Geometry: see drawing. Coordinates: mm, zero at the bounding-box minimum. Give positions to 0.01 mm unless a question says otherwise; leave off trailing zeros. Loops run counter-clockwise (first coordinate to the right, second up) from the corner with the lowest first, then second, coordinate; pieces in that order, holes last. Notation, with made-up numbers: (-17.75, -27) -> (40.25, -27) arc R15 ccw to (40.25, -22) -> close; hole circle Ø8 at (17.5, -20.75). An arc over 180 degrees is marked (long way). Return JSON: item names as keys, results as strings. Group by question number.
(1) Cut plane A-A on y = 16. Return loops of the section in (x, z).
(2) Cut plane C-C on z = 3.25. Return loops of the section in (x, y) (1 decimal).
(3) Cut plane B-B on x = 28.5. Return loops of the section in (y, z), then the cut area to 3 significant figures.
(4) Draft query along Y for the marked faces 1, 2, 3 and 4. Return one class per face: released by +Y, released by -Y, zero draft, split by the parting line, or undercut.
(5) Pin query (flat end, axial travel): pin 1 (5 mm diameter, centred on x = 29.42, y = 13.69, fed in from +Z). Return the tip coordinate at first contact, or that it passes through.
(6) Ray query, line 1 (X direction, y = 12, z = 13.25) (1 decimal); line 2 (X direction, y = 12.25, z = 9) (1 decimal); line 3 (X direction, y = 9.75, z = 15.5) (1 decimal). Return the intervals inside material, ascending. Write a range as from..to.
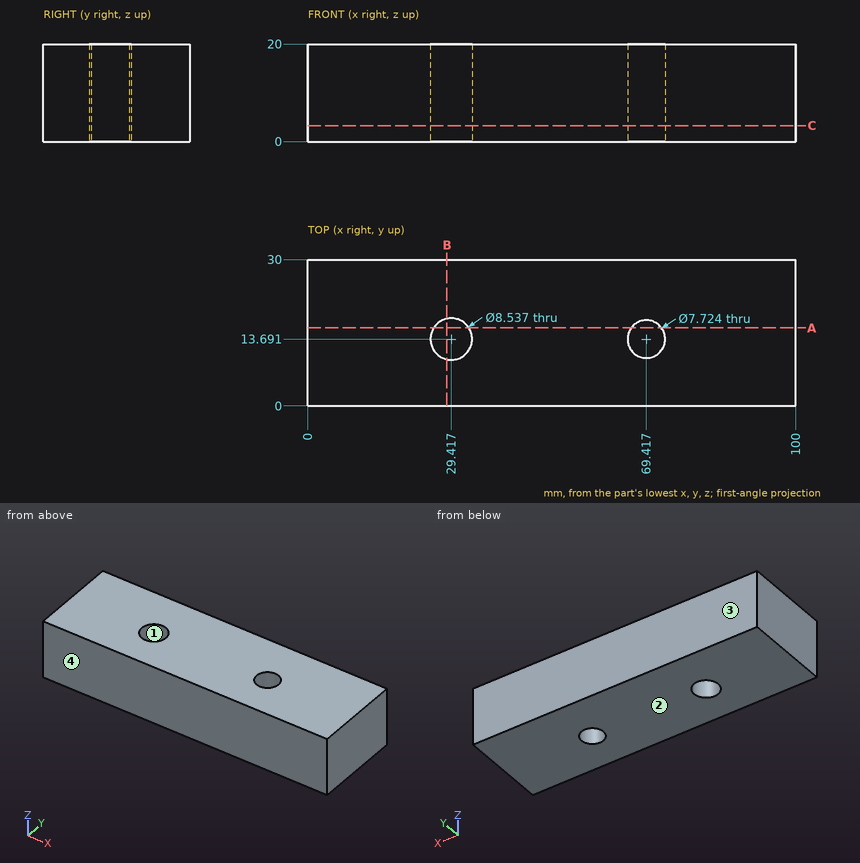
Answers:
{
 "1": {"outline": "(0, 0) -> (25.83, 0) -> (25.83, 20) -> (0, 20) -> close; (33.01, 0) -> (66.32, 0) -> (66.32, 20) -> (33.01, 20) -> close; (72.51, 0) -> (100, 0) -> (100, 20) -> (72.51, 20) -> close"},
 "2": {"outline": "(0, 0) -> (100, 0) -> (100, 30) -> (0, 30) -> close; hole circle Ø8.5 at (29.4, 13.7); hole circle Ø7.7 at (69.4, 13.7)"},
 "3": {"outline": "(0, 0) -> (9.52, 0) -> (9.52, 20) -> (0, 20) -> close; (17.86, 0) -> (30, 0) -> (30, 20) -> (17.86, 20) -> close", "area": "433 mm²"},
 "4": {"face 1": "undercut", "face 2": "zero draft", "face 3": "released by +Y", "face 4": "released by -Y"},
 "5": {"pin 1": "through"},
 "6": {"line 1": "0..25.5, 33.3..65.9, 72.9..100", "line 2": "0..25.4, 33.4..65.8, 73..100", "line 3": "0..27.8, 31.1..100"}
}
